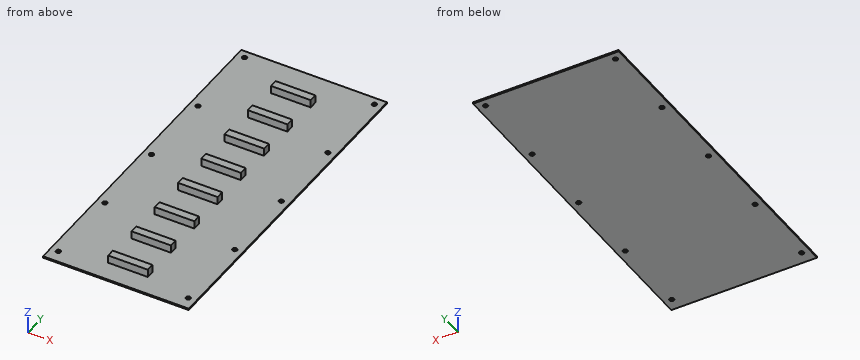
from build123d import *

# Parameters (mm, degrees)
SKETCH1_W                 = 92
SKETCH1_H                 = 213
BOSS_EXTRUDE1_DEPTH       = 1
SKETCH2_W                 = 25
SKETCH2_H                 = 5
BOSS_EXTRUDE2_DEPTH       = 5
F_4_CLEARANCE_HOLE1_D     = 2.9464
F_4_CLEARANCE_HOLE1_DEPTH = 3.175
F_4_CLEARANCE_HOLE1_TIP   = 0.885187864


with BuildPart() as part:
    # Sketch1 → Boss-Extrude1 (new body)
    with BuildSketch(Plane.XY):
        Rectangle(SKETCH1_W, SKETCH1_H)
    extrude(amount=BOSS_EXTRUDE1_DEPTH)

    # Sketch2 → Boss-Extrude2 (add)
    with BuildSketch(Plane.XY.offset(1)):
        with Locations((0, 84)):
            Rectangle(SKETCH2_W, SKETCH2_H)
        with Locations((0, 59)):
            Rectangle(SKETCH2_W, SKETCH2_H)
        with Locations((0, 34)):
            Rectangle(SKETCH2_W, SKETCH2_H)
        with Locations((0, 9)):
            Rectangle(SKETCH2_W, SKETCH2_H)
        with Locations((0, -16)):
            Rectangle(SKETCH2_W, SKETCH2_H)
        with Locations((0, -41)):
            Rectangle(SKETCH2_W, SKETCH2_H)
        with Locations((0, -66)):
            Rectangle(SKETCH2_W, SKETCH2_H)
        with Locations((0, -91)):
            Rectangle(SKETCH2_W, SKETCH2_H)
    extrude(amount=BOSS_EXTRUDE2_DEPTH)

    # #4 Clearance Hole1
    with Locations(Plane.XY.offset(1)):
        with Locations((-41, 101.5), (41, 101.5), (-41, 51.5), (41, 51.5), (-41, 1.5), (41, 1.5), (-41, -48.5), (41, -48.5), (-41, -98.5), (41, -98.5)):
            Hole(F_4_CLEARANCE_HOLE1_D / 2, depth=F_4_CLEARANCE_HOLE1_DEPTH)
            with Locations((0, 0, -(F_4_CLEARANCE_HOLE1_DEPTH + F_4_CLEARANCE_HOLE1_TIP / 2))):  # 118° drill point
                Cone(0, F_4_CLEARANCE_HOLE1_D / 2, F_4_CLEARANCE_HOLE1_TIP, mode=Mode.SUBTRACT)


solid = part.part
Geometry: final body of the model. Coordinates: model frame, mm. Give positions to 0.01 mm unless a question says otherwise; leave off trailing zeros. Write each loop counter-clockwise with the first axis right and the second up, starting at its lowest first coordinate (ties: lowest second). Pieces come first, ordered by that corner, then holes. Notation, with made-up numbers: (51, 3.5) -> (71, 3.5) arc R29 ccw to (71, 26.5) -> close; hole circle Ø4 at (28.5, -17.75). An arc over 180 degrees is marked (long way). Answer in a Markdown table with one row per item.
(1) Section query B-B on x = 24. Return loops of the section in (y, z).
Answers below:
| item | result |
|---|---|
| outline | (-106.5, 0) -> (106.5, 0) -> (106.5, 1) -> (-106.5, 1) -> close |
(2) Pin query (flat end, axial travel): pin 1 (2.5 mm diameter, centred on x = 5, z = 3, fed in from -Y); pin 2 (1 mm diameter, centred on x = -12.5, z = 3, fed in from +Y); pin 3 (2.5 mm diameter, centred on x = 41, y = 51.5, fed in from +Z); pin 4 (2.5 mm diameter, centred on y = -66.5, z = 4, fed in from -X). Return the tip coordinate at first contact, or that it passes through.
Answers below:
| item | result |
|---|---|
| pin 1 | y = -93.5 |
| pin 2 | y = 86.5 |
| pin 3 | through |
| pin 4 | x = -12.5 |
(3) Section query C-C on y = -60.5. Return loops of the section in (x, z).
Answers below:
| item | result |
|---|---|
| outline | (-46, 0) -> (46, 0) -> (46, 1) -> (-46, 1) -> close |
(4) Ray query, line 1 along X through (y, z) = (-98.5, 0.3); line 2 along Y through (x, z) = (41, 0.45); line 3 along Z through (x, y) = (34, 81). Return the intervals inside material, ascending. Write a range as [from, to].
Answers below:
| item | result |
|---|---|
| line 1 | [-46, -42.47], [-39.53, 39.53], [42.47, 46] |
| line 2 | [-106.5, -99.97], [-97.03, -49.97], [-47.03, 0.03], [2.97, 50.03], [52.97, 100.03], [102.97, 106.5] |
| line 3 | [0, 1] |
(5) Section query A-A on z = 2.75. State how many separate pieces and enclosed holes the cut face has, then the cut area to 3 significant figures.
Answers below:
| item | result |
|---|---|
| separate pieces | 8 |
| enclosed holes | 0 |
| area | 1,000 mm^2 |
